```python
from build123d import *

# Parameters (mm, degrees)
F0_W     = 1600
F0_H     = 120
F1_DEPTH = 24
F2_R     = 4.006659
F2_R_2   = 4
F3_DEPTH = 27
F4_R     = 4
F5_DEPTH = 27
F6_W     = 1600
F6_H     = 20
F7_DEPTH = 24


with BuildPart() as f1:
    # F0 (on Front) → F1 (new body)
    with BuildSketch(Plane.XZ):
        Rectangle(F0_W, F0_H)
    extrude(amount=F1_DEPTH)

    # F2 (on face) → F3 (cut)
    with BuildSketch(Plane.YZ.offset(800)):
        with Locations((-10, 40)):
            Circle(F2_R)
        with Locations((-10, -40)):
            Circle(F2_R_2)
    extrude(amount=-F3_DEPTH, mode=Mode.SUBTRACT)

    # F4 (on face) → F5 (cut)
    with BuildSketch(Plane(origin=(-800, 0, 0), x_dir=(0, -1, 0), z_dir=(-1, 0, 0))):
        with Locations((14, 40.100251)):
            Circle(F4_R)
        with Locations((14, -40)):
            Circle(F4_R)
    extrude(amount=-F5_DEPTH, mode=Mode.SUBTRACT)

    # F6 (on face) → F7 (join)
    with BuildSketch(Plane(origin=(0, 0, 0), x_dir=(-1, 0, 0), z_dir=(0, 1, 0))):
        with Locations((0, -50)):
            Rectangle(F6_W, F6_H)
    extrude(amount=F7_DEPTH)


solid = f1.part
```
Design review of the part built by this model. Coordinates are the model's own, in mm. A direction names the side the tool comes from. Coordinates: 2 decimals unless noted, no trailing zeros. Loops run counter-clockwise (first coordinate to the right, second up) from the corner with the lowest first, then second, coordinate; pieces in that order, holes last. Notation, with made-up numbers: (8, 64.25) - (59, 64.25) arc R25 cw to (59, 95.25) - close; hole circle Ø5 at (11, 54). An arc over 180 degrees is marked (long way). Use CSV: the item, a comma, the result in double quotes. Start each with the question number.
1) Tool access review of faces 1 (the flat face through (-11, -24, 1)), 2 (the flat face through (-11, 0, 11)): name each direction out of +Z, -Z, +X, -X, +Y, -Y from which nothing blocks a thin tool from reaching the whole face with its end or side.
2) Consider section A-A on x = 632.5. Write out the cut boundary in (y, z).
3) For pin 1 Ø2.5 at (y, z) = (-13.5, 39) entering from -X; pin 2 Ø13 at (y, z) = (-10, 40) entering from +X; pin 3 Ø8 at (x, y) = (627, 17) entering from +Z; pin 4 Ø6 at (x, z) = (-374, 4.5) entering from +Y, all flat-tipped, find the tip position at first contact; note any pin that passes through.
4) Consider section B-B on y = 11. Write out the cut boundary in (x, z).
5) Consider section C-C on z = -13. Write out the cut boundary in (x, y), then the cut area to 3 significant figures.
6) Wall thickness on L1, parallel to Z at x = 784.25, y = -10; L2, parallel to Z at x = -781.5, y = -14; L3, parallel to Y at x = 354.5, z = -34.5: over which ranges is each line inside the solid? List them lowest first. Write a range as from..to.
Geometry says:
1,face 1,"+Z, -Z, +X, -X, -Y"
1,face 2,"+Z, +X, -X, +Y"
2,outline,"(-24, -60) - (24, -60) - (24, -40) - (0, -40) - (0, 60) - (-24, 60) - close"
3,pin 1,"x = -773"
3,pin 2,"x = 800"
3,pin 3,"z = -40"
3,pin 4,"y = 0"
4,outline,"(-800, -60) - (800, -60) - (800, -40) - (-800, -40) - close"
5,outline,"(-800, -24) - (800, -24) - (800, 0) - (-800, 0) - close"
5,area,"38,400 mm^2"
6,L1,"-60..-44, -36..35.99, 44.01..60"
6,L2,"-60..-44, -36..36.1, 44.1..60"
6,L3,"-24..0"
